```python
from build123d import *

# Parameters (mm, degrees)
BOSS_EXTRUDE1_DEPTH = 80
SKETCH2_R           = 3
CUT_EXTRUDE1_DEPTH  = 28


with BuildPart() as part:
    # Sketch1 → Boss-Extrude1 (new body)
    with BuildSketch(Plane(origin=(0, 0, 0), x_dir=(1, 0, 0), z_dir=(0, 1, 0))):
        with BuildLine():
            Line((-14.5, 13.5), (14.5, 13.5))
            Line((14.5, 13.5), (14.5, -13.5))
            ThreePointArc((14.5, -13.5), (0, -10.355140872), (-14.5, -13.5))
            Line((-14.5, -13.5), (-14.5, 13.5))
        make_face()
    extrude(amount=BOSS_EXTRUDE1_DEPTH)

    # Sketch2 → Cut-Extrude1 (cut, through all)
    with BuildSketch(Plane(origin=(0, 0, -13.5), x_dir=(-1, 0, 0), z_dir=(0, 0, -1))):
        with Locations((0, 70)):
            Circle(SKETCH2_R)
        with Locations((0, 40)):
            Circle(SKETCH2_R)
        with Locations((0, 10)):
            Circle(SKETCH2_R)
    extrude(amount=-CUT_EXTRUDE1_DEPTH, mode=Mode.SUBTRACT)


solid = part.part
```
Design review of the part built by this model. Coordinates are the model's own, in mm. Coordinates: 2 decimals unless noted, no trailing zeros. Write each loop counter-clockwise with the first axis right and the second up, starting at its lowest first coordinate (ties: lowest second). Pieces come first, ordered by that corner, then holes.
1) Insertion check: pin 1 (5.5 mm diameter, centred on x = 0, y = 40, fed in from -Z); pin 2 (3 mm diameter, centred on x = -7, y = 64.5, fed in from +Z); pin 3 (8 mm diameter, centred on x = 1, y = 59.5, fed in from +Z); pin 4 (7 mm diameter, centred on x = 0, y = 10, fed in from +Z). Each pin has a flat end and moves straight along its axis. Give the tip position at first contact, or say it passes through.
2) Mouldability with a two-part tool opening along X and no side actions: class faces 1 (the cylindrical face through (0.65, 67.07, -1.68)), 2 (the cylindrical face through (3.526, 39.44, 10.533)), 3 (the flat face through (-14.5, 39, 0)), 4 (the flat face through (0, 80, 0)) as +X half, -X half, draft (parallel to the pull), parting line (faces both ways), or undercut.
3) Add section C-C (y = 70). Write out the cut boundary in (x, z), plus the area to 3 significant figures.
4) Add section D-D (z = 11.75). Write out the cut boundary in (x, y).
5) Add section A-A (x = 0). Write out the cut boundary in (y, z), plus the area to 3 significant figures.
6) To check wall thickness, follow L1, parallel to Y at x = 0, z = -1.25; L2, parallel to Y at x = -2.25, z = 0.75; L3, parallel to X at y = 70, z = -10.25. State the ranges of each line that lie inside material, in increasing order.
7) Add section B-B (z = 3.5). Write out the cut boundary in (x, y).
Check result:
1. pin 1: passes through
1. pin 2: stops at z = 11.4
1. pin 3: stops at z = 10.71
1. pin 4: stops at z = 10.53
2. face 1: undercut
2. face 2: undercut
2. face 3: -X half
2. face 4: draft
3. outline: (-14.5, -13.5) - (-3, -13.5) - (-3, 10.48) arc R35 cw to (-14.5, 13.5) - close; (3, -13.5) - (14.5, -13.5) - (14.5, 13.5) arc R35 cw to (3, 10.48) - close
3. area: 578 mm2
4. outline: (-14.5, 0) - (-9.78, 0) - (-9.78, 80) - (-14.5, 80) - close; (9.78, 0) - (14.5, 0) - (14.5, 80) - (9.78, 80) - close
5. outline: (0, -13.5) - (7, -13.5) - (7, 10.36) - (0, 10.36) - close; (13, -13.5) - (37, -13.5) - (37, 10.36) - (13, 10.36) - close; (43, -13.5) - (67, -13.5) - (67, 10.36) - (43, 10.36) - close; (73, -13.5) - (80, -13.5) - (80, 10.36) - (73, 10.36) - close
5. area: 1,480 mm2
6. L1: y = 0 to 7, 13 to 37, 43 to 67, 73 to 80
6. L2: y = 0 to 8.02, 11.98 to 38.02, 41.98 to 68.02, 71.98 to 80
6. L3: x = -14.5 to -3, 3 to 14.5
7. outline: (-14.5, 0) - (14.5, 0) - (14.5, 80) - (-14.5, 80) - close; hole circle Ø6 at (0, 10); hole circle Ø6 at (0, 40); hole circle Ø6 at (0, 70)
